Here's how the part is built. I have some questions about the finished solid (model axes, mm). A direction names the side the tool comes from. Give positions to 0.01 mm unless a question says otherwise; leave off trailing zeros. Order: outer loops, then holes, each group sorted by start corner. A loop starts at its lowest first (then second) coordinate and runs counter-clockwise, first axis right, second up. Notation, with made-up numbers: M 84,-11 L 143,-11 A28 cw 143,23 Z; hole C -26.75,68 d4. An arc over 180 degrees is marked long. One line per item, written item: value. Start each with the question number.
from build123d import *

# Parameters (mm, degrees)
EXTRUDE1_DEPTH    = 43.18
SKETCH2_OUTSIDE_W = 27.934
SKETCH2_OUTSIDE_H = 25.958
SKETCH2_OUTSIDE_R = 4.7625
EXTRUDE2_DEPTH    = 38.1


with BuildPart() as part:
    # Sketch1 → Extrude1 (new body)
    with BuildSketch(Plane.XY):
        Polygon((4.244335179, 6.944596596), (-3.892029482, 7.148000386), (-8.136364661, 0.203403789), (-4.244335179, -6.944596596), (3.892029482, -7.148000386), (8.136364661, -0.203403789), align=None)
    extrude(amount=EXTRUDE1_DEPTH)

    # Sketch2 outside → Extrude2 (cut)
    with BuildSketch(Plane.XY.offset(43.18)):
        Rectangle(SKETCH2_OUTSIDE_W, SKETCH2_OUTSIDE_H)
        Circle(SKETCH2_OUTSIDE_R, mode=Mode.SUBTRACT)
    extrude(amount=-EXTRUDE2_DEPTH, mode=Mode.SUBTRACT)


solid = part.part
Item 1: I want a section at B-B on y = 1.5. Write out the boundary of the cut face in (x, z).
Item 2: For faces 1 (the face through (0, 0, 0)), 2 (the face through (4, 3, 5.08)), which set-ups out of +Z, -Z, +X, -X, +Y, -Y let a thin tool reach every point of the face, with its end or its side?
Item 3: I want a section at C-C on z = 27. Write out the boundary of the cut face in (x, y) (1 decimal).
Item 4: I want a section at D-D on x = -5.5. Write out the boundary of the cut face in (y, z).
Item 5: I want a section at A-A on x = 3.25. Write out the boundary of the cut face in (y, z).
Item 6: Please list where these lines run through material, in increasing order: probe 1 along X at (y, z) = (0.25, 18); probe 2 along Z at (x, y) = (-3.5, -5.5); probe 3 along X at (y, z) = (-2.75, 24). Write a range as [from, to].
Item 7: Will these pins go through, and if not, where does the flat tip stop? P1, Ø1, axis at x = -5.5, y = 4, coming from the +Z side; P2, Ø1, axis at x = -4, z = 22.5, coming from the +Y side; P3, Ø5, axis at y = 1, z = 32, coming from the +X side.
Answer below:
1. outline: M -7.34,0 L 7.21,0 L 7.21,5.08 L 4.52,5.08 L 4.52,43.18 L -4.52,43.18 L -4.52,5.08 L -7.34,5.08 Z
2. face 1: -Z, +X, -X, +Y, -Y
2. face 2: +Z
3. outline: C 0,0 d9.5
4. outline: M -4.64,0 L 4.52,0 L 4.52,5.08 L -4.64,5.08 Z
5. outline: M -7.13,0 L 6.97,0 L 6.97,5.08 L 3.48,5.08 L 3.48,43.18 L -3.48,43.18 L -3.48,5.08 L -7.13,5.08 Z
6. probe 1: x = [-4.76, 4.76]
6. probe 2: z = [0, 5.08]
6. probe 3: x = [-3.89, 3.89]
7. P1: stops at z = 5.08
7. P2: stops at y = 3.23
7. P3: stops at x = 4.76
